Design review of the part built by this model. Coordinates are the model's own, in mm. A direction names the side the tool comes from. Coordinates: 2 decimals unless noted, no trailing zeros. Write each loop counter-clockwise with the first axis right and the second up, starting at its lowest first coordinate (ties: lowest second). Pieces come first, ordered by that corner, then holes. Notation, with made-up numbers: (-11, 49.5) - (-3, 49.5) arc R20 cw to (-3, 65.5) - close; hole circle Ø8 at (-34, 28). An arc over 180 degrees is marked (long way). Use a Markdown table: item, result.
from build123d import *

# Parameters (mm, degrees)
SKETCH1_R                                       = 60.5
BOSS_EXTRUDE1_DEPTH                             = 7
SKETCH6_R                                       = 3.5
CUT_EXTRUDE2_DEPTH                              = 70
CUT_EXTRUDE7_DEPTH                              = 10
SKETCH23_W                                      = 42.472377856
SKETCH23_H                                      = 49.728625228
CUT_EXTRUDE8_DEPTH                              = 4
SKETCH24_W                                      = 49.728625228
SKETCH24_H                                      = 1.127718677
CUT_EXTRUDE10_DEPTH                             = 1
CSK_FOR_M2_FLAT_HEAD_MACHINE_SCREW1_D           = 2.4
CSK_FOR_M2_FLAT_HEAD_MACHINE_SCREW1_CSINK_D     = 4.4
CSK_FOR_M2_FLAT_HEAD_MACHINE_SCREW1_CSINK_ANGLE = 90
SKETCH30_W                                      = 24.590301857
SKETCH30_H                                      = 22.033921334
CUT_EXTRUDE11_DEPTH                             = 10
SKETCH39_R                                      = 2.5
CUT_EXTRUDE14_DEPTH                             = 13
SKETCH42_R                                      = 4.5
CUT_EXTRUDE15_DEPTH                             = 1.5
SKETCH43_W                                      = 2.738349456
SKETCH43_H                                      = 1.372281323
CUT_EXTRUDE17_DEPTH                             = 1


with BuildPart() as part:
    # Sketch1 → Boss-Extrude1 (new body)
    with BuildSketch(Plane(origin=(0, 0, 0), x_dir=(0, 1, 0), z_dir=(0, 0, 1))):
        with Locations(Location((0, 0, 0), (0, 0, 270))):
            Circle(SKETCH1_R)
    extrude(amount=BOSS_EXTRUDE1_DEPTH)

    # Sketch6 → Cut-Extrude2 (cut)
    with BuildSketch(Plane(origin=(0, 60.5, -6), x_dir=(-1, 0, 0), z_dir=(0, 1, 0))):
        with Locations((0, 6)):
            Circle(SKETCH6_R)
    extrude(amount=-CUT_EXTRUDE2_DEPTH, mode=Mode.SUBTRACT)

    # Sketch21 → Cut-Extrude7 (cut)
    with BuildSketch(Plane.XY.offset(7)):
        with BuildLine():
            Line((8.487846034, 59.901639958), (8.487846034, -28.542105861))
            Line((8.487846034, -28.542105861), (-53.344148629, -28.542105861))
            ThreePointArc((-53.344148629, -28.542105861), (113.000185213, -78.999671309), (8.487846034, 59.901639958))
        make_face()
    extrude(amount=-CUT_EXTRUDE7_DEPTH, mode=Mode.SUBTRACT)

    # Sketch23 → Cut-Extrude8 (cut)
    with BuildSketch(Plane(origin=(0, 0, 0), x_dir=(1, 0, 0), z_dir=(0, 0, -1))):
        with Locations((-23.236188928, -12.625963158)):
            Rectangle(SKETCH23_W, SKETCH23_H)
    extrude(amount=-CUT_EXTRUDE8_DEPTH, mode=Mode.SUBTRACT)

    # Sketch24 → Cut-Extrude10 (cut)
    with BuildSketch(Plane(origin=(-2, 0, 0), x_dir=(0, -1, 0), z_dir=(-1, 0, 0))):
        with Locations((-12.625963158, 3.436140662)):
            Rectangle(SKETCH24_W, SKETCH24_H)
    extrude(amount=-CUT_EXTRUDE10_DEPTH, mode=Mode.SUBTRACT)

    # CSK for M2 Flat Head Machine Screw1 (through all)
    with Locations(Plane.YX.offset(-4)):
        with Locations((-4.307531, -17.373644116), (5.192468135, -17.377696999), (21.926905074, -17.371512218), (31.426905074, -17.371512218)):
            CounterSinkHole(CSK_FOR_M2_FLAT_HEAD_MACHINE_SCREW1_D / 2, CSK_FOR_M2_FLAT_HEAD_MACHINE_SCREW1_CSINK_D / 2, counter_sink_angle=CSK_FOR_M2_FLAT_HEAD_MACHINE_SCREW1_CSINK_ANGLE)

    # Sketch30 → Cut-Extrude11 (cut)
    with BuildSketch(Plane(origin=(0, 0, 4), x_dir=(1, 0, 0), z_dir=(0, 0, -1))):
        with Locations((-32.177226928, -26.473315105)):
            Rectangle(SKETCH30_W, SKETCH30_H)
        Polygon((-19.882075999, -12.713705866), (-44.472377856, -12.713705866), (-44.472377856, 9.50080752), (-19.871510792, 9.50080752), align=None)
    extrude(amount=-CUT_EXTRUDE11_DEPTH, mode=Mode.SUBTRACT)

    # Sketch39 → Cut-Extrude14 (cut)
    with BuildSketch(Plane(origin=(0, -9.5, 0), x_dir=(-1, 0, 0), z_dir=(0, 1, 0))):
        Circle(SKETCH39_R)
    extrude(amount=-CUT_EXTRUDE14_DEPTH, mode=Mode.SUBTRACT)

    # Sketch42 → Cut-Extrude15 (cut, symmetric)
    with BuildSketch(Plane(origin=(0, -15.738349456, 0), x_dir=(-1, 0, 0), z_dir=(0, 1, 0))):
        Circle(SKETCH42_R)
    extrude(amount=CUT_EXTRUDE15_DEPTH, both=True, mode=Mode.SUBTRACT)

    # Sketch43 → Cut-Extrude17 (cut)
    with BuildSketch(Plane(origin=(-2, 0, 0), x_dir=(0, -1, 0), z_dir=(-1, 0, 0))):
        with Locations((10.869174728, 2.186140662)):
            Rectangle(SKETCH43_W, SKETCH43_H)
    extrude(amount=-CUT_EXTRUDE17_DEPTH, mode=Mode.SUBTRACT)


solid = part.part
(1) For L1, parallel to X at y = 1, z = 6.5; L2, parallel to Y at x = -26, z = 5; L3, parallel to X at y = 28.5, z = 6.75, list the stretches that pass through material, from the lowest coordinate up. Write a range as from..to.
Determined:
| item | result |
|---|---|
| L1 | -60.49..-44.47, -19.88..8.49 |
| L2 | -28.54..-9.5, 12.71..15.46, 37.49..54.63 |
| L3 | -53.37..-44.47, -19.88..8.49 |
(2) Take a section at A-A on y = 0.5. Write out the cut boundary in (x, z), and give its area (3 significant figures).
Determined:
| item | result |
|---|---|
| outline | (-60.5, 0) - (-44.47, 0) - (-44.47, 7) - (-60.5, 7) - close; (-19.88, 4) - (-1, 4) - (-1, 3.35) arc R3.5 cw to (3.5, 0) - (8.49, 0) - (8.49, 7) - (-19.88, 7) - close |
| area | 222 mm2 |
(3) Take a section at B-B on x = -36. Write out the cut boundary in (y, z), and give its area (4 significant figures).
Determined:
| item | result |
|---|---|
| outline | (-28.54, 0) - (-12.24, 0) - (-12.24, 4) - (-9.5, 4) - (-9.5, 7) - (-28.54, 7) - close; (12.71, 4) - (15.46, 4) - (15.46, 7) - (12.71, 7) - close; (37.49, 0) - (48.62, 0) - (48.62, 7) - (37.49, 7) - close |
| area | 208.5 mm2 |
(4) For pin 1 (21.5 mm diameter, centred on x = -17, y = 7.5, fed in from -Z); pin 2 (1 mm diameter, centred on x = 1.5, z = 1, fed in from +Y); pin 3 (1.4 mm diameter, centred on x = -17.37, y = 31.43, fed in from +Z); pin 4 (3 mm diameter, centred on x = -17.38, y = 5.19, fed in from -Z), all flat-tipped, find the tip position at first contact; note any pin that passes through.
Determined:
| item | result |
|---|---|
| pin 1 | z = 4 |
| pin 2 | y = -22.5 |
| pin 3 | through |
| pin 4 | z = 4.7 |
(5) Draft analysis for pull direction Y (two halves, no side actions). For faces 4 (the flat face through (-19, 7, 7)), 5 (the flat face through (-22, -28.542, 4)), 6 (the cylindrical face through (-16.36, -4.95, 6.01)), state which applies: +Y half, -Y half, draft (parallel to the pull), parting line (faces both ways), or undercut.
Determined:
| item | result |
|---|---|
| face 4 | draft |
| face 5 | -Y half |
| face 6 | undercut |
(6) Take a section at D-D on y = 46. Write out the cut boundary in (x, z), and give its area (3 significant figures).
Determined:
| item | result |
|---|---|
| outline | (-39.3, 0) - (-3.5, 0) arc R3.5 cw to (3.5, 0) - (8.49, 0) - (8.49, 7) - (-39.3, 7) - close |
| area | 315 mm2 |
(7) Take a section at C-C on x = 0. Write out the cut boundary in (y, z), and give its area (3 significant figures).
Determined:
| item | result |
|---|---|
| outline | (-28.54, 0) - (-22.5, 0) - (-22.5, 2.5) - (-17.24, 2.5) - (-17.24, 4.5) - (-14.24, 4.5) - (-14.24, 2.5) - (-9.5, 2.5) - (-9.5, 3.5) - (60.5, 3.5) - (60.5, 7) - (-28.54, 7) - close |
| area | 340 mm2 |
(8) Machinability: for faces 1 (the cylindrical face through (-0.1, -15.7, 4.5)), 2 (the flat face through (-32, 12.714, 5)), 3 (the flat face through (0, -22.5, 1)), which of the approach directions +Z, -Z, +X, -X, +Y, -Y give a long, thin tool a straight path to every point of the face, cutting with its end or side? Answer none if there is none.
Determined:
| item | result |
|---|---|
| face 1 | -Z |
| face 2 | +Z, -Z |
| face 3 | -Z, +Y |
